CAD build for the part. Positions are in the model's coordinates, mm. Round coordinates to 2 decimals unless told otherwise and drop trailing zeros. Order: outer loops, then holes, each group sorted by start corner. A loop starts at its lowest first (then second) coordinate and runs counter-clockwise, first axis right, second up. Notation, with made-up numbers: (3.25, 14) -> (52.25, 14) arc R24 ccw to (52.25, 38) -> close; hole circle Ø6 at (-8, 40). An arc over 180 degrees is marked (long way). Return JSON: item names as keys, results as strings. Group by question number.
Q1. Cut at D-D (x = 75). Write the cut outline in (y, z), then the cut area to 3 significant figures.
Q2. Cut at A-A (y = 984.5). Write the cut outline in (x, z), then the cut area to 3 significant figures.
Q3. Flat gauge pins, fed straight in: pin 1 (0.5 mm diameter, centred on y = 987.5, z = 0.5, fed in from +X); pin 2 (0.8 mm diameter, centred on y = 956.5, z = 0.5, fed in from -X). Where does each tip first touch, or does it go through?
Q4. Probe line 1 along X through (y, z) = (983, 1.1); line 2 along X through (y, z) = (995.5, 1.3); line 3 along X through (y, z) = (991.5, 1.25). List the from-to ranges inside material, lowest first.
Q5. Cut at B-B (x = 30). Write the cut outline in (y, z), then the cut area to 3 significant figures.
Q6. Cut at C-C (z = 1.2). Count the separate pieces of the cut face and the enclosed holes in it, then the cut area to 3 significant figures.
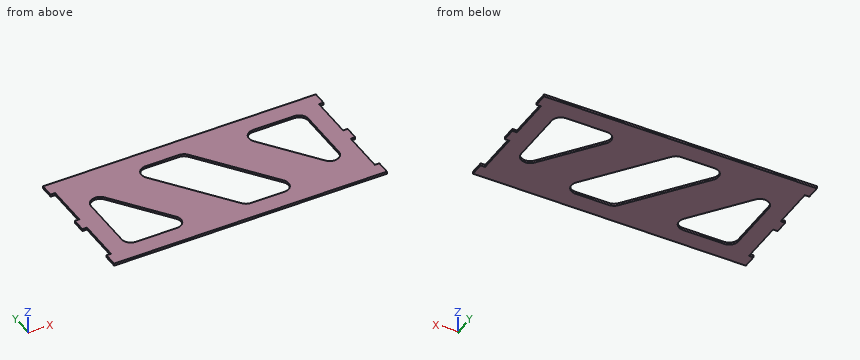
from build123d import *

# Parameters (mm, degrees)
SKETCH1_W           = 183.656
SKETCH1_H           = 88.9
BOSS_EXTRUDE1_DEPTH = 1.5875
CUT_EXTRUDE1_DEPTH  = 1.5875
FILLET1_R           = 6.35
SKETCH3_W           = 1.5875
SKETCH3_H           = 9.525
BOSS_EXTRUDE2_DEPTH = 3.175


with BuildPart() as part:
    # Sketch1 → Boss-Extrude1 (new body)
    with BuildSketch(Plane.XY):
        with Locations((3.944, 974.412014871)):
            Rectangle(SKETCH1_W, SKETCH1_H)
    extrude(amount=BOSS_EXTRUDE1_DEPTH)

    # Sketch2 → Cut-Extrude1 (cut)
    with BuildSketch(Plane.XY.offset(1.5875)):
        with BuildLine():
            Line((-63.754, 990.922014871), (-35.179, 952.822014871))
            ThreePointArc((-35.179, 952.822014871), (-34.579387337, 946.172208539), (-40.259, 942.662014871))
            Line((-40.259, 942.662014871), (-68.834, 942.662014871))
            ThreePointArc((-68.834, 942.662014871), (-73.324128061, 944.52188681), (-75.184, 949.012014871))
            Line((-75.184, 949.012014871), (-75.184, 987.112014871))
            ThreePointArc((-75.184, 987.112014871), (-70.842046314, 993.136153813), (-63.754, 990.922014871))
        make_face()
        with BuildLine():
            Line((71.642, 957.902014871), (43.067, 996.002014871))
            ThreePointArc((43.067, 996.002014871), (42.467387337, 1002.651821202), (48.147, 1006.162014871))
            Line((48.147, 1006.162014871), (76.722, 1006.162014871))
            ThreePointArc((76.722, 1006.162014871), (81.212128061, 1004.302142931), (83.072, 999.812014871))
            Line((83.072, 999.812014871), (83.072, 961.712014871))
            ThreePointArc((83.072, 961.712014871), (78.730046314, 955.687875928), (71.642, 957.902014871))
        make_face()
        Polygon((-39.46525, 1006.162014871), (8.15975, 942.662014871), (47.35325, 942.662014871), (-0.27175, 1006.162014871), align=None)
    extrude(amount=-CUT_EXTRUDE1_DEPTH, mode=Mode.SUBTRACT)

    # Fillet1
    fillet1_edges = [part.edges().sort_by_distance(p)[0] for p in [
        (8.15975, 942.662014871, 0.79375),
        (-39.46525, 1006.162014871, 0.79375),
        (-0.27175, 1006.162014871, 0.79375),
        (47.35325, 942.662014871, 0.79375),
    ]]
    fillet(fillet1_edges, radius=FILLET1_R)

    # Sketch3 → Boss-Extrude2 (add)
    with BuildSketch(Plane(origin=(95.772, 0, 0), x_dir=(0, 0, -1), z_dir=(1, 0, 0))):
        with Locations((-0.79375, 1014.099514871)):
            Rectangle(SKETCH3_W, SKETCH3_H)
        with Locations((-0.79375, 934.724514871)):
            Rectangle(SKETCH3_W, SKETCH3_H)
        with Locations((-0.79375, 974.412014871)):
            Rectangle(SKETCH3_W, SKETCH3_H)
    boss_extrude2 = extrude(amount=BOSS_EXTRUDE2_DEPTH)

    # Mirror2: Boss-Extrude2 across plane
    add(boss_extrude2.mirror(Plane(origin=(3.944, 0, 0), x_dir=(0, 0, 1), z_dir=(1, 0, 0))))


solid = part.part
Solution:
{
 "1": {"outline": "(929.96, 0) -> (955.6, 0) -> (955.6, 1.59) -> (929.96, 1.59) -> close; (1006.16, 0) -> (1018.86, 0) -> (1018.86, 1.59) -> (1006.16, 1.59) -> close", "area": "60.9 mm²"},
 "2": {"outline": "(-87.88, 0) -> (-75.18, 0) -> (-75.18, 1.59) -> (-87.88, 1.59) -> close; (-58.94, 0) -> (-23.22, 0) -> (-23.22, 1.59) -> (-58.94, 1.59) -> close; (15.97, 0) -> (51.69, 0) -> (51.69, 1.59) -> (15.97, 1.59) -> close; (83.07, 0) -> (95.77, 0) -> (95.77, 1.59) -> (83.07, 1.59) -> close", "area": "154 mm²"},
 "3": {"pin 1": "stops at x = 95.77", "pin 2": "stops at x = -87.88"},
 "4": {"line 1": "x = -87.88 to -75.18, -57.81 to -22.09, 17.1 to 52.82, 83.07 to 95.77", "line 2": "x = -87.88 to -31.47, 7.72 to 43.44, 83.07 to 95.77", "line 3": "x = -87.88 to -73.42, -64.24 to -28.47, 10.72 to 46.44, 83.07 to 95.77"},
 "5": {"outline": "(929.96, 0) -> (942.66, 0) -> (942.66, 1.59) -> (929.96, 1.59) -> close; (965.8, 0) -> (1018.86, 0) -> (1018.86, 1.59) -> (965.8, 1.59) -> close", "area": "104 mm²"},
 "6": {"separate pieces": "1", "enclosed holes": "3", "area": "11,300 mm²"}
}
